Autodesk Inventor part; units mm, degrees
ref_plane "作業平面1" through (0, 0, 0.15) normal (0, 0, 1) x (1, 0, 0)
ref_plane "YZ Plane" through (0, 0, 0) normal (1, 0, 0) x (0, 1, 0)
ref_plane "XZ Plane" through (0, 0, 0) normal (0, 1, 0) x (-1, 0, 0)
ref_plane "作業平面1" through (0, 0, 0.15) normal (0, 0, 1) x (1, 0, 0)
sketch "スケッチ1" plane through (0, 0, 0.15) normal (0, 0, 1) x (1, 0, 0)
  line L0 (0, -24) -> (-27.3, -24)
  line L1 (-3.7, -24) -> (-3.7, -10.5)
  line L2 (-3.7, -10.5) -> (4.3, -10.5)
  line L3 (6.3, -8.5) -> (6.3, 1.5)
  line L4 (6.3, 1.5) -> (1.3, 1.5)
  line L5 (-27.3, 0) -> (0, 0)
  line L6 (1.3, 1.5) -> (1.3, 0)
  circle A0 centre (-6, -21.7) radius 1.25
  circle A1 centre (-19, -21.7) radius 1.25
  circle A2 centre (-6, -21.7) radius 2.3 construction
  circle A3 centre (-19, -21.7) radius 2.3 construction
  line L7 (1.3, 0) -> (0, 0)
  line L8 (-21.3, -24) -> (-21.3, 0)
  circle A4 centre (-6, -2.3) radius 1.25
  circle A5 centre (-19, -2.3) radius 1.25
  line L9 (1.3, 0) -> (0.8, 0)
  arc A6 (0.3, 0) -> (1.3, 0) centre (0.8, 0) ccw
  line L10 (-6, -21.7) -> (-19, -21.7)
  line L11 (-19, -21.7) -> (-19, -2.3)
  line L12 (-19, -2.3) -> (-6, -2.3)
  line L13 (-6, -2.3) -> (-6, -21.7)
  arc A7 (-6, -19.4) -> (-8.3, -21.7) centre (-6, -21.7) ccw
  arc A8 (-16.7, -21.7) -> (-19, -19.4) centre (-19, -21.7) ccw
  arc A9 (-19, -4.6) -> (-16.7, -2.3) centre (-19, -2.3) ccw
  arc A10 (-8.3, -2.3) -> (-6, -4.6) centre (-6, -2.3) ccw
  arc A11 (4.3, -10.5) -> (6.3, -8.5) centre (4.3, -8.5) ccw
  line L14 (-3.5, -2) -> (0.3, -2)
  line L15 (1.3, -3) -> (1.3, -8)
  line L16 (0.3, -9) -> (-3.5, -9)
  line L17 (-4.5, -8) -> (-4.5, -3)
  arc A12 (0.3, -9) -> (1.3, -8) centre (0.3, -8) ccw
  arc A13 (1.3, -3) -> (0.3, -2) centre (0.3, -3) ccw
  arc A14 (-3.5, -2) -> (-4.5, -3) centre (-3.5, -3) ccw
  arc A15 (-4.5, -8) -> (-3.5, -9) centre (-3.5, -8) ccw
  arc A16 (-4.5, -4.0436) -> (-3.7196, -2) centre (-6, -2.3) ccw
  line L18 (-3.7, -10.5) -> (-21.3, -10.5)
  line L19 (-3.5, -9) -> (-21.3, -9)
  point P0 (6.3, -10.5)
  point P1 (0.8, -0.5)
  point P2 (-3.7167, -2.0238)
  point P3 (-6, -9)
  point P4 (-19, -9)
  dimension "d0" = 1.5
  dimension "d1" = 12
  dimension "d2" = 10
  dimension "d3" = 5
  dimension "d9" = 0.5
  dimension "d13" = 2
  dimension "d14" = 1
  dimension "d15" = 1.5
  dimension "d16" = 1.5
  dimension "d17" = 5
  dimension "d18" = 1.5
extrude "押し出し1" add sketch "スケッチ1" along normal blind 4 contours L18 L13 A4 L12 A5 L11 L19 L8 L5 L7 A6 L6 L4 L3 A11 L2 | L8 L19 L11 L18 | L18 L11 L19 L13 | A10 L12 A4 L13 | L11 A5 L12 A9 | L17 A14 A16
sketch "スケッチ2" plane through (1.3, 1.5, 0.15) normal (0, 1, 0) x (1, 0, 0)
  line L0 (5, 0) -> (5, -4)
  line L1 (0, 0) -> (-22.6, 0)
  line L2 (5, -4) -> (0, 0) construction
  circle A0 centre (2.5, -2) radius 1.1
  point P0 (-1.3, 0.15)
  dimension "d6" = 2.2
extrude "押し出し2" cut sketch "スケッチ2" against normal blind 5
fillet "フィレット1" radius 2 9 edges at (-19, -4.6, 2.15) (-16.7, -2.3, 2.15) (-8.3, -2.3, 2.15) (-6, -4.6, 2.15) (-4.5, -4.0436, 2.15) (-3.7167, -2.0238, 2.15) (-19, -9, 2.15) (-6, -9, 2.15) (-21.3, -10.5, 2.15)
sketch "スケッチ3" plane through (0, 0, 0.15) normal (0, 0, -1) x (-1, 0, 0)
  line L0 (21.3, 0) -> (21.3, -8.5)
  line L1 (-0.3, 0) -> (21.3, 0)
  arc A0 (-1.3, 0) -> (-0.3, 0) centre (-0.8, 0) ccw
  line L2 (-1.3, 1.5) -> (-1.3, 0)
  line L3 (-6.3, 1.5) -> (-1.3, 1.5)
  line L4 (-6.3, -8.5) -> (-6.3, 1.5)
  arc A1 (-6.3, -8.5) -> (-4.3, -10.5) centre (-4.3, -8.5) ccw
  line L5 (19.3, -10.5) -> (-4.3, -10.5)
  circle A2 centre (6, -2.3) radius 1.25
  arc A3 (9.8066, -2.3) -> (8.0361, -3.3698) centre (9.8066, -4.3) ccw
  line L6 (15.1934, -2.3) -> (9.8066, -2.3)
  arc A4 (16.9639, -3.3698) -> (15.1934, -2.3) centre (15.1934, -4.3) ccw
  arc A5 (16.9639, -3.3698) -> (17.9302, -4.3361) centre (19, -2.3) ccw
  arc A6 (19, -6.1066) -> (17.9302, -4.3361) centre (17, -6.1066) ccw
  line L7 (19, -7) -> (19, -6.1066)
  line L8 (6, -6.1066) -> (6, -7)
  arc A7 (7.0698, -4.3361) -> (6, -6.1066) centre (8, -6.1066) ccw
  arc A8 (7.0698, -4.3361) -> (8.0361, -3.3698) centre (6, -2.3) ccw
  circle A9 centre (19, -2.3) radius 1.25
  line L9 (2.0503, -2) -> (-0.3, -2)
  arc A10 (3.8874, -3.2093) -> (4.1279, -3.6361) centre (6, -2.3) ccw
  line L10 (4.5, -8) -> (4.5, -4.798)
  arc A11 (3.5, -9) -> (4.5, -8) centre (3.5, -8) ccw
  line L11 (-0.3, -9) -> (3.5, -9)
  arc A12 (-1.3, -8) -> (-0.3, -9) centre (-0.3, -8) ccw
  line L12 (-1.3, -3) -> (-1.3, -8)
  arc A13 (-0.3, -2) -> (-1.3, -3) centre (-0.3, -3) ccw
  arc A14 (3.8874, -3.2093) -> (2.0503, -2) centre (2.0503, -4) ccw
  arc A15 (4.5, -4.798) -> (4.1279, -3.6361) centre (2.5, -4.798) ccw
  line L13 (8, -9) -> (17, -9)
  arc A16 (6, -7) -> (8, -9) centre (8, -7) ccw
  arc A17 (17, -9) -> (19, -7) centre (17, -7) ccw
  arc A18 (19.3, -10.5) -> (21.3, -8.5) centre (19.3, -8.5) ccw
  point P0 (0, 0)
extrude "押し出し3" [suppressed]
properties part number "SolenoidMount"
Build history of the part. All positions in model axes, mm. A direction names the side the tool comes from. Give positions to 0.01 mm unless a question says otherwise; leave off trailing zeros. Loops run counter-clockwise (first coordinate to the right, second up) from the corner with the lowest first, then second, coordinate; pieces in that order, holes last.
Item 1: Slice it at B-B, the plane y = -1.5. List the corners of the cut face in (x, z), and give its area (3 significant figures).
Answers follow:
outline: (-21.3, 0.15) - (-19.96, 0.15) - (-19.96, 4.15) - (-21.3, 4.15) - close; (-18.04, 0.15) - (-6.96, 0.15) - (-6.96, 4.15) - (-18.04, 4.15) - close; (-5.04, 0.15) - (6.3, 0.15) - (6.3, 4.15) - (-5.04, 4.15) - close; hole circle Ø2.2 at (3.8, 2.15)
area: 91.2 mm2
Item 2: Drill centre lines: line 1 (X direction, y = -6.5, z = 1.55); line 2 (Z direction, x = 3.8, y = 0); line 3 (X direction, y = -2.75, z = 1.2). Where is each one in solid material? Low to high.
Answers follow:
line 1: x = -21.3 to -19, -6 to -4.5, 1.3 to 6.3
line 2: z = 0.15 to 1.05, 3.25 to 4.15
line 3: x = -21.3 to -20.17, -17.83 to -16.46, -8.54 to -7.17, -4.83 to -3.61, 1.27 to 3.25, 4.35 to 6.3
Item 3: Which spindle directions (+Z, -Z, +X, -X, +Y, -Y) get a long thin tool onto all of the face, cutting with end or side? Do faces 4 (the face through (-4.199, -8.715, 2.122)), 5 (the face through (-5, -4, 4.15)), 6 (the face through (4, -3.5, 2)). Say none if no direction does.
Answers follow:
face 4: +Z, -Z
face 5: +Z, +X, -X, +Y, -Y
face 6: +Y
Item 4: Slice it at A-A, the plane x = -1.75. List the corners of the cut face in (y, z).
Answers follow:
outline: (-10.5, 0.15) - (-9, 0.15) - (-9, 4.15) - (-10.5, 4.15) - close; (-2, 0.15) - (0, 0.15) - (0, 4.15) - (-2, 4.15) - close
Item 5: Flat gauge pin, fed straight in: pin 1 (1 mm diameter, centred on x = -9.5, z = 2, fed in from +Y). Where does the tip first touch, or does it go through?
Answers follow:
pin 1: stops at y = 0
Item 6: Slice it at C-C, the plane z = 2.15. Give the number of separate pieces and of enclosed holes in the cut face, and give its area (3 significant figures).
Answers follow:
separate pieces: 1
enclosed holes: 4
area: 160 mm2
Item 7: Pull direction Y, two halves, no side cores. Call faces 1 (the face through (-17.37, -3.92, 2.12)), 2 (the face through (-11, 0, 2)), 3 (the face through (1.3, 1, 2)): released by +Y, released by -Y, zero draft, split by the parting line, or undercut.
Answers follow:
face 1: undercut
face 2: released by +Y
face 3: zero draft
Item 8: Slice it at D-D, the plane x = 3.8. List the corners of the cut face in (y, z).
Answers follow:
outline: (-10.5, 0.15) - (1.5, 0.15) - (1.5, 1.05) - (-3.5, 1.05) - (-3.5, 3.25) - (1.5, 3.25) - (1.5, 4.15) - (-10.5, 4.15) - close
